from build123d import *

# Parameters (mm, degrees)
F1_DEPTH = 1.5
F3_DEPTH = 25


with BuildPart() as f1:
    # F0 (on Right) → F1 (new body, symmetric)
    with BuildSketch(Plane.YZ):
        with BuildLine():
            Line((0, 6.685786), (0, 0))
            Line((0, 0), (0.5, 0))
            Line((0.5, 0), (0.5, 6.892786))
            ThreePointArc((0.5, 6.892786), (0.42388, 7.27547), (0.207107, 7.599893))
            Line((0.207107, 7.599893), (-3.807107, 11.614107))
            ThreePointArc((-3.807107, 11.614107), (-4.02388, 11.93853), (-4.1, 12.321214))
            Line((-4.1, 12.321214), (-4.1, 35.5))
            ThreePointArc((-4.1, 35.5), (-3.807107, 36.207107), (-3.1, 36.5))
            Line((-3.1, 36.5), (11.336, 36.5))
            Line((11.336, 36.5), (11.336, 37))
            Line((11.336, 37), (-3.6, 37))
            ThreePointArc((-3.6, 37), (-4.307107, 36.707107), (-4.6, 36))
            Line((-4.6, 36), (-4.6, 12.114214))
            ThreePointArc((-4.6, 12.114214), (-4.52388, 11.73153), (-4.307107, 11.407107))
            Line((-4.307107, 11.407107), (-0.292893, 7.392893))
            ThreePointArc((-0.292893, 7.392893), (-0.07612, 7.06847), (0, 6.685786))
        make_face()
    extrude(amount=F1_DEPTH, both=True)

    # F2 (on face) → F3 (cut)
    with BuildSketch(Plane.XY.offset(37)):
        with BuildLine():
            ThreePointArc((-1.5, 9.336), (-1.081139, 10.560745), (0, 11.272492))
            ThreePointArc((0, 11.272492), (1.081139, 10.560745), (1.5, 9.336))
            Line((1.5, 9.336), (1.5, 11.336))
            Line((1.5, 11.336), (-1.5, 11.336))
            Line((-1.5, 11.336), (-1.5, 9.336))
        make_face()
    extrude(amount=-F3_DEPTH, mode=Mode.SUBTRACT)


solid = f1.part
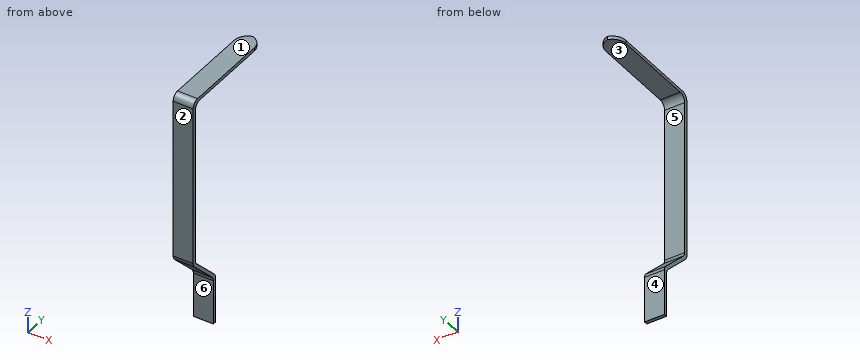
Model file for the job. Use its own axes, mm. Face numbers are marked on the shaded views. A direction names the side the tool comes from. Round coordinates to 2 decimals unless told otherwise and drop trailing zeros. Loops run counter-clockwise (first coordinate to the right, second up) from the corner with the lowest first, then second, coordinate; pieces in that order, holes last.
1. Band-saw the part on B-B, the plane z = 23.5. List the corners of the cut face in (x, y).
Check values:
outline: (-1.5, -4.6) - (1.5, -4.6) - (1.5, -4.1) - (-1.5, -4.1) - close
2. Drop flat-ended pins along their axis: P1, Ø0.9, axis at x = -0.5, y = 3, coming from the -Z side; P2, Ø2, axis at y = 1, z = 9.5, coming from the +X side; P3, Ø0.9, axis at x = 0, z = 27.5, coming from the +Y side; P4, Ø1.5, axis at x = 0.5, z = 4.5, coming from the -Y side. Give the stop position or say it passes through.
Check values:
P1: stops at z = 36.5
P2: passes through
P3: stops at y = -4.1
P4: stops at y = 0
3. Band-saw the part on C-C, the plane x = -1.15. List the corners of the cut face in (y, z).
Check values:
outline: (-4.6, 12.11) arc R1 ccw to (-4.31, 11.41) - (-0.29, 7.39) arc R1 cw to (0, 6.69) - (0, 0) - (0.5, 0) - (0.5, 6.89) arc R1 ccw to (0.21, 7.6) - (-3.81, 11.61) arc R1 cw to (-4.1, 12.32) - (-4.1, 35.5) arc R1 cw to (-3.1, 36.5) - (10.47, 36.5) - (10.47, 37) - (-3.6, 37) arc R1 ccw to (-4.6, 36) - close
4. Mould opens along Z. For the marked faces 1, 2 and 3 say: +Z half, -Z half, draft (parallel to the pull), parting line (faces both ways), or undercut.
Check values:
face 1: +Z half
face 2: draft
face 3: undercut
5. Band-saw the part on D-D, the plane y = 6. List the corners of the cut face in (x, z).
Check values:
outline: (-1.5, 36.5) - (1.5, 36.5) - (1.5, 37) - (-1.5, 37) - close
6. Wall check: probe 1 along Z at (x, y) = (0.45, 4.25); probe 2 along Y at (x, z) = (-0.05, 34.5); probe 3 along Y at (x, z) = (-1.2, 5.5). Give the ranges that are in metal, low to high.
Check values:
probe 1: z = 36.5 to 37
probe 2: y = -4.6 to -4.1
probe 3: y = 0 to 0.5
7. Tool access for the marked faces 4, 5 and 6: list every direction of +Z, -Z, +X, -X, +Y, -Y with a clear straight run to the whole face (end or side of a thin tool).
Check values:
face 4: -Z, +X, -X, +Y
face 5: +X, -X, +Y
face 6: -Z, +X, -X, -Y
8. Band-saw the part on A-A, the plane y = -2. List the corners of the cut face in (x, z).
Check values:
outline: (-1.5, 9.1) - (1.5, 9.1) - (1.5, 9.81) - (-1.5, 9.81) - close; (-1.5, 36.5) - (1.5, 36.5) - (1.5, 37) - (-1.5, 37) - close
